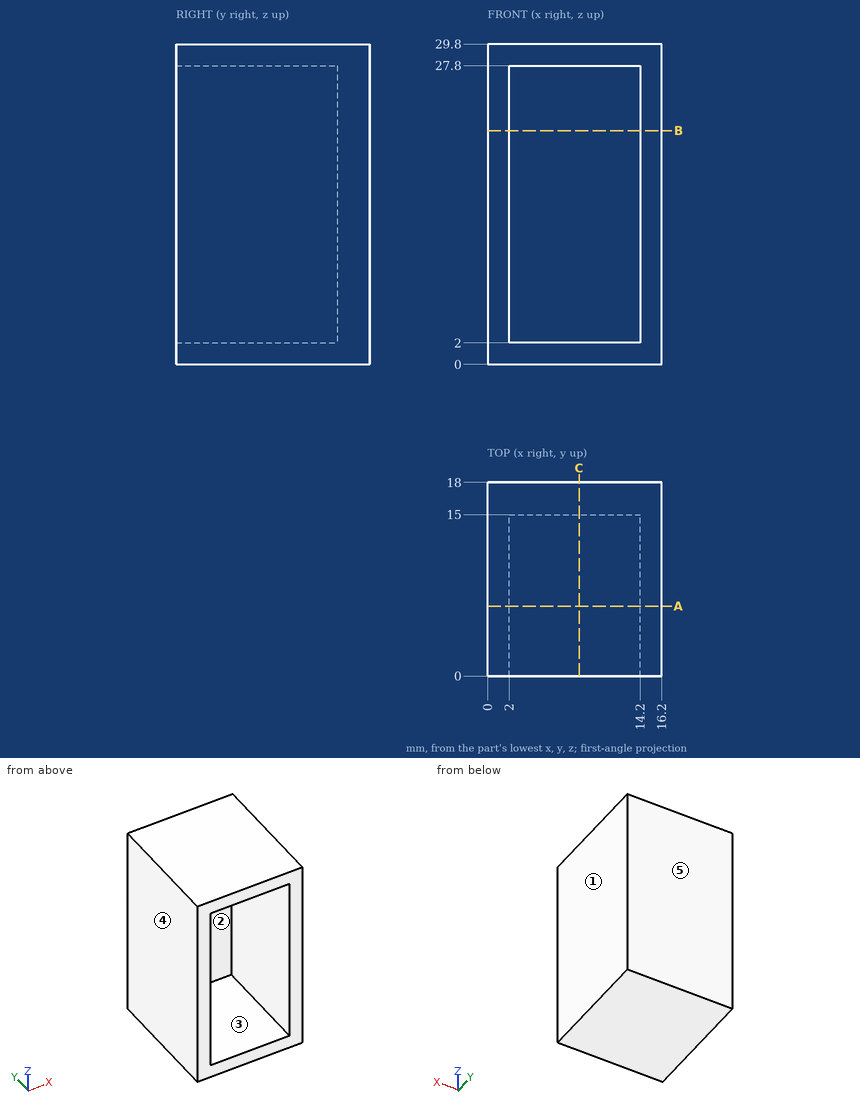
Here's the drawing with two shaded views (mm, measured from the low corner). I have some questions. A direction names the side the tool comes from. Coordinates: 2 decimals unless noted, no trailing zeros. Order: outer loops, then holes, each group sorted by start corner. A loop starts at its lowest first (then second) coordinate and runs counter-clockwise, first axis right, second up. Notation, with made-up numbers: (51.25, 76) -> (70.25, 76) arc R19 ccw to (70.25, 84) -> close; hole circle Ø1 at (-23.5, 8.25). An arc over 180 degrees is marked (long way). Write each question's results on one line, items separated by ' | '.
Item 1: Which directions (+Z, -Z, +X, -X, +Y, -Y) give clear straight access to the entire face, cutting with the end or side of a thin tool? Please do the marked faces 1 and 2.
Results are:
face 1: +Z, -Z, +X, +Y, -Y | face 2: -Y
Item 2: If I drill on line 1 along Z through (x, y) = (10, 3.75); line 2 along X through (y, z) = (13.5, 2.5); line 3 along Y through (x, z) = (13.25, 8.25), over which ranges is the centre line in solid material (lowest first)?
Results are:
line 1: 0 to 2, 27.8 to 29.8 | line 2: 0 to 2, 14.2 to 16.2 | line 3: 15 to 18
Item 3: I want a section at B-B, the plane z = 21.75. Write out the boundary of the cut face in (x, y), then the cut area to 3 significant figures.
Results are:
outline: (0, 0) -> (2, 0) -> (2, 15) -> (14.2, 15) -> (14.2, 0) -> (16.2, 0) -> (16.2, 18) -> (0, 18) -> close | area: 109 mm²
Item 4: If we mould it in two halves opening along X, with no side actions, what happens to the marked faces 3, 4 and 5? For each: +X half, -X half, draft (parallel to the pull), parting line (faces both ways), or undercut.
Results are:
face 3: undercut | face 4: -X half | face 5: draft
Item 5: I want a section at A-A, the plane y = 6.5. Write out the boundary of the cut face in (x, z), then the cut area to 3 significant figures.
Results are:
outline: (0, 0) -> (16.2, 0) -> (16.2, 29.8) -> (0, 29.8) -> close; hole (2, 2) -> (14.2, 2) -> (14.2, 27.8) -> (2, 27.8) -> close | area: 168 mm²
Item 6: I want a section at C-C, the plane x = 8.5. Write out the boundary of the cut face in (y, z).
Results are:
outline: (0, 0) -> (18, 0) -> (18, 29.8) -> (0, 29.8) -> (0, 27.8) -> (15, 27.8) -> (15, 2) -> (0, 2) -> close
